```python
from build123d import *

# Parameters (mm, degrees)
SKETCH1_W               = 34.5
SKETCH1_H               = 20
BOSS_EXTRUDE1_DEPTH     = 2
SKETCH2_W               = 26.4
SKETCH2_H               = 2.2
SKETCH2_W_2             = 2.5
SKETCH2_H_2             = 16
SKETCH2_H_3             = 8.4
BOSS_EXTRUDE2_DEPTH     = 10
CUT_EXTRUDE1_DEPTH      = 17.5
CUT_EXTRUDE1_DEPTH_BACK = 17.5
SKETCH3_W               = 3
SKETCH3_H               = 4
CUT_EXTRUDE2_DEPTH      = 10
FILLET1_R               = 2
BOSS_EXTRUDE3_DEPTH     = 5
SKETCH7_W               = 34.5
SKETCH7_H               = 20
CUT_EXTRUDE3_DEPTH      = 2


with BuildPart() as part:
    # Sketch1 → Boss-Extrude1 (new body)
    with BuildSketch(Plane.XY):
        Rectangle(SKETCH1_W, SKETCH1_H)
    extrude(amount=BOSS_EXTRUDE1_DEPTH)

    # Sketch2 → Boss-Extrude2 (add)
    with BuildSketch(Plane.XY):
        Polygon((-17.25, 10), (17.25, 10), (17.25, 8), (17.25, -8), (17.25, -10), (-17.25, -10), align=None)
        with Locations((-2.05, 6.9)):
            Rectangle(SKETCH2_W, SKETCH2_H, mode=Mode.SUBTRACT)
        with Locations((-2.05, -6.9)):
            Rectangle(SKETCH2_W, SKETCH2_H, mode=Mode.SUBTRACT)
        with Locations((14, 0)):
            Rectangle(SKETCH2_W_2, SKETCH2_H_2, mode=Mode.SUBTRACT)
        with Locations((-2.05, 0)):
            Rectangle(SKETCH2_W, SKETCH2_H_3, mode=Mode.SUBTRACT)
    extrude(amount=BOSS_EXTRUDE2_DEPTH)

    # Sketch3 → Cut-Extrude1 (cut, two sides: drawn at the far end of the back side and taken through both)
    with BuildSketch(Plane(origin=(0, 0, 0), x_dir=(0, 0, -1), z_dir=(1, 0, 0)).offset(-CUT_EXTRUDE1_DEPTH_BACK)):
        with Locations((-3.5, 0)):
            Rectangle(SKETCH3_W, SKETCH3_H)
    extrude(amount=CUT_EXTRUDE1_DEPTH + CUT_EXTRUDE1_DEPTH_BACK, mode=Mode.SUBTRACT)

    # Sketch4 → Cut-Extrude2 (cut)
    with BuildSketch(Plane(origin=(0, 10, 0), x_dir=(1, 0, 0), z_dir=(0, 1, 0))):
        with BuildLine():
            Line((-7.35, -9.1875), (-7.35, -11.2875))
            Line((-7.35, -11.2875), (-3.15, -11.2875))
            Line((-3.15, -11.2875), (-3.15, -9.1875))
            ThreePointArc((-3.15, -9.1875), (-5.25, -7.0875), (-7.35, -9.1875))
        make_face()
    extrude(amount=-CUT_EXTRUDE2_DEPTH, mode=Mode.SUBTRACT)

    # Fillet1
    fillet1_edges = [part.edges().sort_by_distance(p)[0] for p in [
        (0, -10, 0),
        (0, 10, 0),
    ]]
    fillet(fillet1_edges, radius=FILLET1_R)

    # Sketch6 → Boss-Extrude3 (add)
    with BuildSketch(Plane(origin=(0, 10, 0), x_dir=(1, 0, 0), z_dir=(0, 1, 0))):
        Polygon((-7.75, -2), (-2.75, -2), (-2.75, -4), (-4.5, -4), (-4.5, -6), (-6, -6), (-6, -4), (-7.75, -4), align=None)
    extrude(amount=-BOSS_EXTRUDE3_DEPTH)

    # Sketch7 → Cut-Extrude3 (cut)
    with BuildSketch(Plane.XY):
        Rectangle(SKETCH7_W, SKETCH7_H)
    extrude(amount=CUT_EXTRUDE3_DEPTH, mode=Mode.SUBTRACT)


solid = part.part
```
CAD build for the part. Positions are in the model's coordinates, mm. A direction names the side the tool comes from. Round coordinates to 2 decimals unless told otherwise and drop trailing zeros. Order: outer loops, then holes, each group sorted by start corner. A loop starts at its lowest first (then second) coordinate and runs counter-clockwise, first axis right, second up. Notation, with made-up numbers: (25.25, 74) - (73.25, 74) arc R9 cw to (73.25, 79) - close; hole circle Ø10 at (35, -18). An arc over 180 degrees is marked (long way). Answer as CSV lines item,"result". Start each with the question number.
1. Saw through at A-A, the plane y = 6.5. Write the cut outline in (x, z).
2. Saw through at B-B, the plane x = -5.25. Write the cut outline in (y, z).
3. Pin check, flat tips, straight feed: pin 1 (1.3 mm diameter, centred on x = 12, y = 0, fed in from -Z); pin 2 (1.6 mm diameter, centred on x = -5.5, y = 7, fed in from +Z). Stop position of each tip, or through.
4. Pull direction Y, two halves, no side cores. Call faces 1 (the face through (-2, -8, 6)), 2 (the face through (14, 8, 6)), 3 (the face through (-7.35, 5, 9.6)), 4 (the face through (0, 10, 6)): +Y half, -Y half, draft (parallel to the pull), parting line (faces both ways), or undercut.
5. Saw through at C-C, the plane z = 4.5. Count the separate pieces of the cut face and the enclosed holes in it, and give its area (3 significant figures).
6. Drill centre lines: L1, parallel to X at y = -3.5, z = 4.5; L2, parallel to Y at x = 11, z = 6; L3, parallel to Y at x = 15, z = 2.75. Where is each one in solid material? Low to high. Write a range as [from, to].
7. Saw through at D-D, the plane x = 12. Write the cut outline in (y, z).
8. Tool access for faces 5 (the face through (12, 0, 5)), 6 (the face through (-5.2, 9.01, 7.09)), 7 (the face through (-5, 7, 6)), 8 (the face through (11.15, -7, 6)): list every direction of +Z, -Z, +X, -X, +Y, -Y with a clear straight run to the whole face (end or side of a thin tool).
Model answer:
1,outline,"(-17.25, 2) - (-15.25, 2) - (-15.25, 10) - (-17.25, 10) - close; (-7.75, 2) - (-2.75, 2) - (-2.75, 4) - (-4.5, 4) - (-4.5, 6) - (-6, 6) - (-6, 4) - (-7.75, 4) - close; (11.15, 2) - (12.75, 2) - (12.75, 10) - (11.15, 10) - close; (15.25, 2) - (17.25, 2) - (17.25, 10) - (15.25, 10) - close"
2,outline,"(-10, 2) - (-8, 2) - (-8, 10) - (-10, 10) - close; (-5.8, 2) - (-4.2, 2) - (-4.2, 10) - (-5.8, 10) - close; (4.2, 2) - (10, 2) - (10, 7.09) - (8, 7.09) - (8, 6) - (5.8, 6) - (5.8, 7.09) - (4.2, 7.09) - close"
3,pin 1,"stops at z = 5"
3,pin 2,"stops at z = 6"
4,face 1,"undercut"
4,face 2,"undercut"
4,face 3,"draft"
4,face 4,"+Y half"
5,separate pieces,"2"
5,enclosed holes,"3"
5,area,"293 mm²"
6,L1,"x = [-17.25, -15.25], [11.15, 12.75], [15.25, 17.25]"
6,L2,"y = [-10, -8], [-5.8, -4.2], [4.2, 5.8], [8, 10]"
6,L3,"y = [-10, -8], [8, 10]"
7,outline,"(-10, 2) - (-2, 2) - (-2, 5) - (2, 5) - (2, 2) - (10, 2) - (10, 10) - (-10, 10) - close"
8,face 5,"-Z, +X, -X"
8,face 6,"+Z, +Y"
8,face 7,"+Z"
8,face 8,"+Z, -Z"
